The figure shows three views and two pictorial views of one solid part (mm, origin at its lowest corner). Answer the questions. A direction names the side the tool comes from. Round coordinates to 2 decimals unless told otherwise and drop trailing zeros. Write each loop counter-clockwise with the first axis right and the second up, starting at its lowest first coordinate (ties: lowest second). Pieces come first, ordered by that corner, then holes.
Item 1: A tool of negligible diameter and unlimited length cuts with its end or side. For the marked faces 1, 2 and 3, from which of +Z, -Z, +X, -X, +Y, -Y can it reach the whole face along a straight path? Write none if from no direction.
Item 2: Find section C-C on x = 29. Give the vertices of the cut face in (y, z).
Item 3: Each of these flat-tipped pins is pushed along its axis until it touches: pin 1 (5 mm diameter, centred on x = 69, z = 3, fed in from -Y); pin 2 (6 mm diameter, centred on y = 1.5, z = 14.5, fed in from -X); pin 3 (2.5 mm diameter, centred on x = 29.5, y = 5.5, fed in from +Z); pin 4 (2 mm diameter, centred on y = 5.5, z = 12, fed in from +X). Where does it stop, or does it pass through?
Item 4: Find section A-A on y = 4.75. Give the vertices of the cut face in (x, z).
Item 5: Find section B-B on z = 4.75. Give the vertices of the cut face in (x, y), then the cut area to 3 significant figures.
Item 6: Find the intervals of material crossed by probe 1 along Z at (x, y) = (53.5, 4.5); probe 2 along X at (y, z) = (5, 8.5), in increasing order.
Item 7: Find section D-D on x = 67. Give the vertices of the cut face in (y, z).
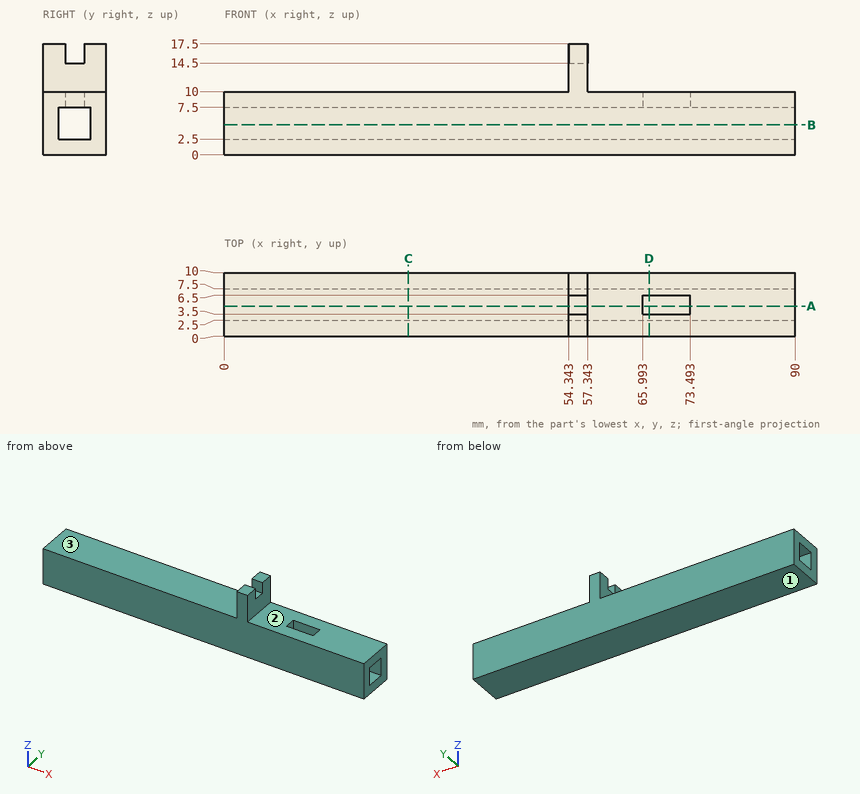
Check values:
1. face 1: -Z, +X, -X, +Y, -Y
1. face 2: +Z, +X, +Y, -Y
1. face 3: +Z, -X, +Y, -Y
2. outline: (0, 0) - (10, 0) - (10, 10) - (0, 10) - close; hole (2.5, 2.5) - (7.5, 2.5) - (7.5, 7.5) - (2.5, 7.5) - close
3. pin 1: stops at y = 0
3. pin 2: stops at x = 54.34
3. pin 3: stops at z = 10
3. pin 4: stops at x = 57.34
4. outline: (0, 0) - (90, 0) - (90, 2.5) - (0, 2.5) - close; (0, 7.5) - (65.99, 7.5) - (65.99, 10) - (57.34, 10) - (57.34, 14.5) - (54.34, 14.5) - (54.34, 10) - (0, 10) - close; (73.49, 7.5) - (90, 7.5) - (90, 10) - (73.49, 10) - close
5. outline: (0, 0) - (90, 0) - (90, 2.5) - (0, 2.5) - close; (0, 7.5) - (90, 7.5) - (90, 10) - (0, 10) - close
5. area: 450 mm2
6. probe 1: z = 0 to 2.5, 7.5 to 10
6. probe 2: x = 0 to 65.99, 73.49 to 90
7. outline: (0, 0) - (10, 0) - (10, 10) - (6.5, 10) - (6.5, 7.5) - (7.5, 7.5) - (7.5, 2.5) - (2.5, 2.5) - (2.5, 7.5) - (3.5, 7.5) - (3.5, 10) - (0, 10) - close
